Geometry: final body of the model. Coordinates: model frame, mm. A direction names the side the tool comes from. Round coordinates to 2 decimals unless told otherwise and drop trailing zeros. Loops run counter-clockwise (first coordinate to the right, second up) from the corner with the lowest first, then second, coordinate; pieces in that order, holes last. Notation, with made-up numbers: (69, 23) -> (108, 23) arc R15 cw to (108, 33) -> close; hole circle Ø9 at (27, -5.75). An arc over 180 degrees is marked (long way). Answer in a Markdown table with one row per item.
```python
from build123d import *

# Parameters (mm, degrees)
SKETCH1_R           = 29.5
SKETCH1_R_2         = 27.1
BOSS_EXTRUDE1_DEPTH = 4
SKETCH1_3_R         = 27.1
SKETCH1_3_R_2       = 12
BOSS_EXTRUDE2_DEPTH = 18
BOSS_EXTRUDE3_START = 9.8
SKETCH1_4_R         = 12
SKETCH1_4_R_2       = 10
BOSS_EXTRUDE3_DEPTH = 3
SKETCH4_R           = 2.15
CUT_EXTRUDE1_DEPTH  = 6


with BuildPart() as part:
    # Sketch1 → Boss-Extrude1 (new body)
    with BuildSketch(Plane.XY):
        Circle(SKETCH1_R)
        Circle(SKETCH1_R_2, mode=Mode.SUBTRACT)
    extrude(amount=BOSS_EXTRUDE1_DEPTH)

    # Sketch1<3> → Boss-Extrude2 (add)
    with BuildSketch(Plane.XY):
        Circle(SKETCH1_3_R)
        Circle(SKETCH1_3_R_2, mode=Mode.SUBTRACT)
    extrude(amount=BOSS_EXTRUDE2_DEPTH)

    # Sketch1<4> → Boss-Extrude3 (add)
    with BuildSketch(Plane.XY.offset(BOSS_EXTRUDE3_START)):
        Circle(SKETCH1_4_R)
        Circle(SKETCH1_4_R_2, mode=Mode.SUBTRACT)
    extrude(amount=BOSS_EXTRUDE3_DEPTH)

    # Sketch4 → Cut-Extrude1 (cut)
    with BuildSketch(Plane.XY.offset(18)):
        with Locations((0, 17.5)):
            Circle(SKETCH4_R)
        with Locations((17.5, 0)):
            Circle(SKETCH4_R)
        with Locations((0, -17.5)):
            Circle(SKETCH4_R)
        with Locations((-17.5, 0)):
            Circle(SKETCH4_R)
    extrude(amount=-CUT_EXTRUDE1_DEPTH, mode=Mode.SUBTRACT)


solid = part.part
```
Item 1: First-contact query: P1, Ø7, axis at x = 0, y = -17.5, coming from the -Z side; P2, Ø1.3, axis at x = -0.5, y = 17, coming from the +Z side; P3, Ø6, axis at x = 20.5, z = 15, coming from the +Y side; P4, Ø4, axis at x = 1, z = 4, coming from the +Y side. Flat tips, straight axial feed; report the tip coordinate or a pass-through.
Ans:
| item | result |
|---|---|
| P1 | z = 0 |
| P2 | z = 12 |
| P3 | y = 20.69 |
| P4 | y = 29.5 |
Item 2: Ray query, L1, parallel to Y at x = 0, z = 14.15; L2, parallel to Y at x = 0, z = 10.9; L3, parallel to Y at x = 0, z = 6.5. Return the intervals inside material, ascending.
Ans:
| item | result |
|---|---|
| L1 | -27.1 to -19.65, -15.35 to -12, 12 to 15.35, 19.65 to 27.1 |
| L2 | -27.1 to -10, 10 to 27.1 |
| L3 | -27.1 to -12, 12 to 27.1 |
Item 3: Section query A-A, the plane y = 0. Output: boundary loops of the cut face in (x, z), and give its area (3 significant figures).
Ans:
| item | result |
|---|---|
| outline | (-29.5, 0) -> (-12, 0) -> (-12, 9.8) -> (-10, 9.8) -> (-10, 12.8) -> (-12, 12.8) -> (-12, 18) -> (-15.35, 18) -> (-15.35, 12) -> (-19.65, 12) -> (-19.65, 18) -> (-27.1, 18) -> (-27.1, 4) -> (-29.5, 4) -> close; (10, 9.8) -> (12, 9.8) -> (12, 0) -> (29.5, 0) -> (29.5, 4) -> (27.1, 4) -> (27.1, 18) -> (19.65, 18) -> (19.65, 12) -> (15.35, 12) -> (15.35, 18) -> (12, 18) -> (12, 12.8) -> (10, 12.8) -> close |
| area | 523 mm2 |
Item 4: Set-up query: faces 4 (the flat face through (0, -13, 0)), 5 (the flat face through (-5, 9, 12.8)), 6 (the cylindrical face through (-11.99, 0.53, 4.83)). Return all of +Z, -Z, +X, -X, +Y, -Y with unobstructed straight access to the full face (end or side cutting, diameter ignored); none if empty.
Ans:
| item | result |
|---|---|
| face 4 | -Z, +X, -X, +Y, -Y |
| face 5 | +Z |
| face 6 | -Z |
Item 5: Section query D-D, the plane z = 8. Output: boundary loops of the cut face in (x, y).
Ans:
| item | result |
|---|---|
| outline | circle Ø54.2 at (0, 0); hole circle Ø24 at (0, 0) |
Item 6: Mould query, pull axis Y, two halves, no side actions, for faces 1 (the cylindrical face through (28.14, 8.86, 1.97)), 2 (the flat face through (6, -12, 18)), 3 (the flat face through (0, -17, 12)). Classes: released by +Y, released by -Y, zero draft, split by the parting line, or undercut.
Ans:
| item | result |
|---|---|
| face 1 | split by the parting line |
| face 2 | zero draft |
| face 3 | undercut |
Item 7: Section query C-C, the plane z = 14.25. Output: boundary loops of the cut face in (x, y), and give its area (3 significant figures).
Ans:
| item | result |
|---|---|
| outline | circle Ø54.2 at (0, 0); hole circle Ø4.3 at (-17.5, 0); hole circle Ø24 at (0, 0); hole circle Ø4.3 at (0, -17.5); hole circle Ø4.3 at (0, 17.5); hole circle Ø4.3 at (17.5, 0) |
| area | 1,800 mm2 |
